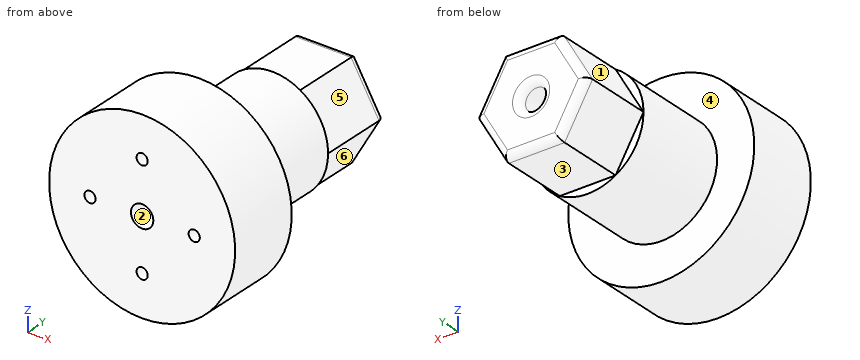
from build123d import *

# Parameters (mm, degrees)
CROQUIS1_R              = 12.5
CROQUIS1_R_2            = 0.75
SALIENTE_EXTRUIR1_DEPTH = 10
CROQUIS2_R              = 7.5
SALIENTE_EXTRUIR2_DEPTH = 13
SALIENTE_EXTRUIR4_START = -1
CROQUIS5_R              = 12.5
SALIENTE_EXTRUIR4_DEPTH = 1
SALIENTE_EXTRUIR3_DEPTH = 10
CROQUIS4_R              = 1.5
CORTAR_EXTRUIR1_DEPTH   = 38.436613095
REDONDEO1_R             = 1


with BuildPart() as part:
    # Croquis1 → Saliente-Extruir1 (new body)
    with BuildSketch(Plane(origin=(0, 0, 0), x_dir=(1, 0, 0), z_dir=(0, 1, 0))):
        with Locations(Location((0, 0, 0), (0, 0, 270))):
            Circle(CROQUIS1_R)
        with Locations(Location((7, 0, 0), (0, 0, 270))):
            Circle(CROQUIS1_R_2, mode=Mode.SUBTRACT)
        with Locations(Location((0, -7, 0), (0, 0, 270))):
            Circle(CROQUIS1_R_2, mode=Mode.SUBTRACT)
        with Locations(Location((-7, 0, 0), (0, 0, 270))):
            Circle(CROQUIS1_R_2, mode=Mode.SUBTRACT)
        with Locations(Location((0, 7, 0), (0, 0, 270))):
            Circle(CROQUIS1_R_2, mode=Mode.SUBTRACT)
    extrude(amount=SALIENTE_EXTRUIR1_DEPTH)

    # Croquis2 → Saliente-Extruir2 (add)
    with BuildSketch(Plane(origin=(0, 10, 0), x_dir=(1, 0, 0), z_dir=(0, 1, 0))):
        with Locations(Location((0, 0, 0), (0, 0, 94.421562439))):
            Circle(CROQUIS2_R)
    extrude(amount=SALIENTE_EXTRUIR2_DEPTH)

    # Croquis5 → Saliente-Extruir4 (add)
    with BuildSketch(Plane(origin=(0, 10, 0), x_dir=(1, 0, 0), z_dir=(0, 1, 0)).offset(SALIENTE_EXTRUIR4_START)):
        with Locations(Location((0, 0, 0), (0, 0, 270))):
            Circle(CROQUIS5_R)
    extrude(amount=SALIENTE_EXTRUIR4_DEPTH)

    # Croquis3 → Saliente-Extruir3 (add)
    with BuildSketch(Plane(origin=(0, 23, 0), x_dir=(1, 0, 0), z_dir=(0, 1, 0))):
        Polygon((7.5, 0), (3.75, 6.495190528), (-3.75, 6.495190528), (-7.5, 0), (-3.75, -6.495190528), (3.75, -6.495190528), align=None)
    extrude(amount=SALIENTE_EXTRUIR3_DEPTH)

    # Croquis4 → Cortar-Extruir1 (cut, through all)
    with BuildSketch(Plane(origin=(0, 33, 0), x_dir=(1, 0, 0), z_dir=(0, 1, 0))):
        with Locations(Location((0, 0, 0), (0, 0, 270))):
            Circle(CROQUIS4_R)
    extrude(amount=-CORTAR_EXTRUIR1_DEPTH, mode=Mode.SUBTRACT)

    # Redondeo1
    redondeo1_edges = [part.edges().sort_by_distance(p)[0] for p in [
        (5.625, 33, 3.247595264),
        (5.625, 33, -3.247595264),
        (0, 33, -6.495190528),
        (-5.625, 33, -3.247595264),
        (-5.625, 33, 3.247595264),
        (0, 33, 6.495190528),
        (0, 33, -1.5),
    ]]
    fillet(redondeo1_edges, radius=REDONDEO1_R)


solid = part.part
Read the model definition and answer for the solid it produces. Units are mm, in the model's axes. Face numbers are marked on the shaded views. A direction names the side the tool comes from. Give positions to 0.01 mm unless a question says otherwise; leave off trailing zeros. Write each loop counter-clockwise with the first axis right and the second up, starting at its lowest first coordinate (ties: lowest second). Pieces come first, ordered by that corner, then holes. Notation, with made-up numbers: (10, 26) -> (33, 26) arc R20 cw to (33, 44) -> close; hole circle Ø2 at (81.5, 73.25). An arc over 180 degrees is marked (long way). Answer as a JSON object with one key per item and string values. Group by question number.
1) Find section B-B (z = 7). Write down the section's boundary in (x, y), and give its area (3 significant figures).
2) Find section C-C (x = -9.25). Write down the section's boundary in (y, z).
3) Find section A-A (x = 0). Write down the section's boundary in (y, z), and give its area (3 significant figures).
4) Consider L1, parallel to X at y = 5.75, z = 0; L2, parallel to Y at x = 8.5, z = -1; L3, parallel to Y at x = 4.5, z = -5.25. Determine where each line is inside the solid, lowest interval first. Write a range as from..to.
5) Each of these flat-tipped pins is pushed along its axis until it touches: P1, Ø1.7, axis at x = 0, z = 7, coming from the +Y side; P2, Ø4, axis at y = 27.5, z = -0.5, coming from the +X side; P3, Ø4, axis at x = 4.5, y = 17, coming from the +Z side. Where does it stop, or does it pass through?
6) Find section D-D (z = 11.25). Write down the section's boundary in (x, y).
7) A tool of negligible diameter and unlimited length cuts with its end or side. For the marked faces 4, 5 and 6, from which of +Z, -Z, +X, -X, +Y, -Y can it reach the whole face along a straight path? Write none if from no direction.
8) The mould has two halves that part along X. Classify the marked faces 1, 2 and 3: +X half, -X half, draft (parallel to the pull), parting line (faces both ways), or undercut.
Values follow:
{
 "1": {"outline": "(-10.36, 0) -> (-0.75, 0) -> (-0.75, 9) -> (0.75, 9) -> (0.75, 0) -> (10.36, 0) -> (10.36, 10) -> (2.69, 10) -> (2.69, 23) -> (-2.69, 23) -> (-2.69, 10) -> (-10.36, 10) -> close", "area": "264 mm2"},
 "2": {"outline": "(0, -8.41) -> (10, -8.41) -> (10, 8.41) -> (0, 8.41) -> close"},
 "3": {"outline": "(0, -12.5) -> (10, -12.5) -> (10, -7.5) -> (23, -7.5) -> (23, -6.5) -> (32, -6.5) arc R1 ccw to (33, -5.5) -> (33, -2.5) arc R1 ccw to (32, -1.5) -> (0, -1.5) -> (0, -6.25) -> (9, -6.25) -> (9, -7.75) -> (0, -7.75) -> close; (0, 1.5) -> (32, 1.5) arc R1 ccw to (33, 2.5) -> (33, 5.5) arc R1 ccw to (32, 6.5) -> (23, 6.5) -> (23, 7.5) -> (10, 7.5) -> (10, 12.5) -> (0, 12.5) -> (0, 7.75) -> (9, 7.75) -> (9, 6.25) -> (0, 6.25) -> close", "area": "448 mm2"},
 "4": {"L1": "x = -12.5..-7.75, -6.25..-1.5, 1.5..6.25, 7.75..12.5", "L2": "y = 0..10", "L3": "y = 0..23"},
 "5": {"P1": "stops at y = 32.76", "P2": "stops at x = 7.5", "P3": "stops at z = 7.07"},
 "6": {"outline": "(-5.45, 0) -> (5.45, 0) -> (5.45, 10) -> (-5.45, 10) -> close"},
 "7": {"face 4": "+Y", "face 5": "+Z, +X, +Y", "face 6": "-Z, +X, +Y"},
 "8": {"face 1": "-X half", "face 2": "undercut", "face 3": "draft"}
}
